from build123d import *

# Parameters (mm, degrees)
SKETCH_1_R          = 19.95169504
EXTRUDE_1_DEPTH     = 100
CUT_EXTRUDE_1_DEPTH = 5


with BuildPart() as part:
    # 草图1 → 凸台-拉伸1 (new body)
    with BuildSketch(Plane(origin=(0, 0, 0), x_dir=(1, 0, 0), z_dir=(0, 1, 0))):
        Circle(SKETCH_1_R)
    extrude(amount=EXTRUDE_1_DEPTH)

    # 草图2 → 切除-拉伸1 (cut)
    with BuildSketch(Plane.XY.offset(19.95169504)):
        with BuildLine():
            Line((-5.839636377, 22.448895044), (-5.839636377, 51.197874129))
            ThreePointArc((-5.839636377, 51.197874129), (0, 57.037510505), (5.839636377, 51.197874129))
            Line((5.839636377, 51.197874129), (5.839636377, 22.448895044))
            ThreePointArc((5.839636377, 22.448895044), (0, 16.609258667), (-5.839636377, 22.448895044))
        make_face()
    extrude(amount=-CUT_EXTRUDE_1_DEPTH, mode=Mode.SUBTRACT)


solid = part.part
Geometry check sheet. Reference: the model listing, model coordinates, mm. A direction names the side the tool comes from. Coordinates: 2 decimals unless noted, no trailing zeros. Loops run counter-clockwise (first coordinate to the right, second up) from the corner with the lowest first, then second, coordinate; pieces in that order, holes last. Notation, with made-up numbers: (27.25, -32) - (50.25, -32) arc R22 cw to (50.25, -12) - close; hole circle Ø1 at (26, 69). An arc over 180 degrees is marked (long way). Use one line per item in the form item = value. Start each with the question number.
Item 1: Section check A-A, the plane x = 0. Enter the section's corners in (y, z), and give its area (3 significant figures).
Item 2: Gauge pin test, flat ends, axial feed: pin 1 (1.5 mm diameter, centred on x = -14.5, y = 74.5, fed in from +Z); pin 2 (1 mm diameter, centred on x = 3, y = 26, fed in from -Z); pin 3 (8 mm diameter, centred on x = -15.5, y = 12.5, fed in from -Z). Record the tip position at first contact, or that the pin passes through.
Item 3: Mould release check, pull along Y, two halves, no side actions. Record for faces 3 (the face through (0.13, 16.61, 17.49)), 4 (the face through (0, 100, 0)), 5 (the face through (0, 0, 0)): +Y half, -Y half, draft (parallel to the pull), parting line (faces both ways), or undercut.
Item 4: Tool access check on faces 1 (the face through (5.84, 37, 17)), 2 (the face through (-2.6, 49.3, -19.78)). Record the directions out of +Z, -Z, +X, -X, +Y, -Y that give a thin tool (end or side, any length) a straight path to the whole face; none if there is none.
Item 5: Section check D-D, the plane y = 83.5. Enter the section's corners in (x, z), and give its area (3 significant figures).
Item 6: Section check B-B, the plane y = 39. Enter the section's corners in (x, z).
Item 7: Thickness scan on probe 1 along Z at (x, y) = (-0.5, 47); probe 2 along X at (y, z) = (26.5, 15); probe 3 along Z at (x, y) = (-7.5, 23.5). Record the ranges inside material, lowest first.
Item 8: Section check C-C, the plane z = -5.5. Enter the section's corners in (x, y), and give its area (3 significant figures).
Computed:
q1.outline = (0, -19.95) - (100, -19.95) - (100, 19.95) - (57.04, 19.95) - (57.04, 14.95) - (16.61, 14.95) - (16.61, 19.95) - (0, 19.95) - close
q1.area = 3,790 mm2
q2.pin_1 = 14.46
q2.pin_2 = -19.79
q2.pin_3 = -16.3
q3.face_3 = undercut
q3.face_4 = +Y half
q3.face_5 = -Y half
q4.face_1 = +Z
q4.face_2 = +Y, -Y
q5.outline = circle Ø39.9 at (0, 0)
q5.area = 1,250 mm2
q6.outline = (-5.84, 14.95) - (-5.84, 19.08) arc R19.95 ccw (long way) to (5.84, 19.08) - (5.84, 14.95) - close
q7.probe_1 = -19.95 to 14.95
q7.probe_2 = -13.16 to -5.84, 5.84 to 13.16
q7.probe_3 = -18.49 to 18.49
q8.outline = (-19.18, 0) - (19.18, 0) - (19.18, 100) - (-19.18, 100) - close
q8.area = 3,840 mm2
